Geometry check sheet. Reference: the model listing, model coordinates, mm. Give positions to 0.01 mm unless a question says otherwise; leave off trailing zeros. Order: outer loops, then holes, each group sorted by start corner. A loop starts at its lowest first (then second) coordinate and runs counter-clockwise, first axis right, second up.
from build123d import *

# Parameters (mm, degrees)
RESSALTO_EXTRUS_O1_DEPTH = 98
CHANFRO1_SIZE            = 2
CORTE_EXTRUS_O1_DEPTH    = 108


with BuildPart() as part:
    # Esboço1 → Ressalto-extrusão1 (new body)
    with BuildSketch(Plane.XY):
        Polygon((0, 0), (-7.610404057, -12.859217835), (-9.331566424, -11.840591257), (-1.721162367, 1.018626578), align=None)
    extrude(amount=RESSALTO_EXTRUS_O1_DEPTH)

    # Chanfro1
    chanfro1_edges = [part.edges().sort_by_distance(p)[0] for p in [
        (-9.331566424, -11.840591257, 49),
    ]]
    chamfer(chanfro1_edges, length=CHANFRO1_SIZE - 0.0001)  # a hair under: the kernel refuses the full size

    # Esboço2 → Corte-extrusão1 (cut)
    with BuildSketch(Plane(origin=(0, 0, 0), x_dir=(-1, 0, 0), z_dir=(0, 0, -1))):
        Polygon((6.735745015, -7.454459757), (7.610404057, -12.859217835), (9.393966164, -10.156838796), align=None)
    extrude(amount=-CORTE_EXTRUS_O1_DEPTH, mode=Mode.SUBTRACT)


solid = part.part
Item 1: Gauge pin test, flat ends, axial feed: pin 1 (3 mm diameter, centred on y = -7, z = 56.5, fed in from +X); pin 2 (2 mm diameter, centred on y = -10.5, z = 16, fed in from -X); pin 3 (2 mm diameter, centred on x = -1.5, z = 68, fed in from -Y). Record the tip position at first contact, or that the pin passes through.
Reported:
pin 1: stops at x = -3.26
pin 2: stops at x = -7.39
pin 3: stops at y = -4.22
Item 2: Sectioned sample at B-B (x = -2.75). Enter the section's corners in (y, z).
Reported:
outline: (-4.65, 0) - (-0.72, 0) - (-0.72, 98) - (-4.65, 98) - close
Item 3: Scan lines: L1, parallel to Y at x = -6, z = 8.5; L2, parallel to X at y = -3.75, z = 36.5; L3, parallel to X at y = -1.75, z = 31.5. Record each from-to range of solid material in increasing order.
Reported:
L1: y = -10.14 to -6.21
L2: x = -4.54 to -2.22
L3: x = -3.36 to -1.04
Item 4: Sectioned sample at A-A (z = 70). Enter the section's corners in (x, y), and give its area (3 significant figures).
Reported:
outline: (-7.61, -12.86) - (0, 0) - (-1.72, 1.02) - (-6.74, -7.45) - close
area: 24.8 mm2
